Check sheet for the modelled part. Datum: model origin and axes. Units: mm. A direction names the side the tool comes from. Round coordinates to 2 decimals unless told otherwise and drop trailing zeros. Order: outer loops, then holes, each group sorted by start corner. A loop starts at its lowest first (then second) coordinate and runs counter-clockwise, first axis right, second up.
```python
from build123d import *

# Parameters (mm, degrees)
SKETCH1_W           = 10
SKETCH1_H           = 10
BOSS_EXTRUDE1_DEPTH = 5
SKETCH2_W           = 3
SKETCH2_H           = 5
CUT_EXTRUDE1_DEPTH  = 13.247448714
SKETCH3_W           = 3
SKETCH3_H           = 3
BOSS_EXTRUDE2_DEPTH = 5
SKETCH4_W           = 2
SKETCH4_H           = 2
BOSS_EXTRUDE3_DEPTH = 2


with BuildPart() as part:
    # Sketch1 → Boss-Extrude1 (new, symmetric)
    with BuildSketch(Plane(origin=(0, 0, 0), x_dir=(1, 0, 0), z_dir=(0, 1, 0))):
        Rectangle(SKETCH1_W, SKETCH1_H)
    extrude(amount=BOSS_EXTRUDE1_DEPTH, both=True)

    # Sketch2 → Cut-Extrude1 (cut, through all)
    with BuildSketch(Plane.XY.offset(5)):
        with Locations((-3.5, 0)):
            Rectangle(SKETCH2_W, SKETCH2_H)
    extrude(amount=-CUT_EXTRUDE1_DEPTH, mode=Mode.SUBTRACT)

    # Sketch3 → Boss-Extrude2 (add)
    with BuildSketch(Plane(origin=(5, 0, 0), x_dir=(0, 0, -1), z_dir=(1, 0, 0))):
        Rectangle(SKETCH3_W, SKETCH3_H)
    extrude(amount=BOSS_EXTRUDE2_DEPTH)

    # Sketch4 → Boss-Extrude3 (add)
    with BuildSketch(Plane(origin=(5, 0, 0), x_dir=(0, 0, -1), z_dir=(1, 0, 0))):
        with Locations((0, 4)):
            Rectangle(SKETCH4_W, SKETCH4_H)
    boss_extrude3 = extrude(amount=BOSS_EXTRUDE3_DEPTH)

    # Mirror1: Boss-Extrude3 across plane
    add(boss_extrude3.mirror(Plane.ZX))


solid = part.part
```
Item 1: Sectioned sample at B-B (y = -1). Record the cut outline in (x, z).
Answer:
outline: (-2, -5) - (5, -5) - (5, -1.5) - (10, -1.5) - (10, 1.5) - (5, 1.5) - (5, 5) - (-2, 5) - close
Item 2: Scan lines: line 1 along Y through (x, z) = (-2.75, -2); line 2 along X through (y, z) = (0.75, -3); line 3 along X through (y, z) = (-1, -1). Record each from-to range of solid material in increasing order.
Answer:
line 1: y = -5 to -2.5, 2.5 to 5
line 2: x = -2 to 5
line 3: x = -2 to 10
Item 3: Release check for a two-part mould opening along Y. For faces 5 (the flat face through (7, 4, 0)), 6 (the flat face through (7, -1.5, 0)), 7 (the flat face through (1, -5, 0)), 8 (the flat face through (1, 5, 0)) record: released by +Y, released by -Y, zero draft, split by the parting line, or undercut.
Answer:
face 5: zero draft
face 6: undercut
face 7: released by -Y
face 8: released by +Y
Item 4: Access from +Z, -Z, +X, -X, +Y, -Y to the whole of each face (thin tool, end or side, straight path). Record for faces 1 (the flat face through (6, 4, 1)), 2 (the flat face through (7, 0, -1.5)), 3 (the flat face through (7, 0, 1.5)), 4 (the flat face through (7, 1.5, 0)).
Answer:
face 1: +Z, +X, +Y
face 2: -Z, +X, +Y, -Y
face 3: +Z, +X, +Y, -Y
face 4: +Z, -Z, +X
Item 5: Go/stop test with flat-tipped pins: P1, Ø1.5, axis at x = 7, y = 0.5, coming from the +Z side; P2, Ø4, axis at y = 1, z = -1, coming from the -X side; P3, Ø1, axis at y = -3.5, z = 0.5, coming from the +X side; P4, Ø2.5, axis at x = 8, y = -0.5, coming from the -Z side. Record where each tip stops, or that it passes through.
Answer:
P1: stops at z = 1.5
P2: stops at x = -5
P3: stops at x = 7
P4: stops at z = -1.5
Item 6: Sectioned sample at D-D (z = 0.75). Record the cut outline in (x, y).
Answer:
outline: (-5, -5) - (7, -5) - (7, -3) - (5, -3) - (5, -1.5) - (10, -1.5) - (10, 1.5) - (5, 1.5) - (5, 3) - (7, 3) - (7, 5) - (-5, 5) - (-5, 2.5) - (-2, 2.5) - (-2, -2.5) - (-5, -2.5) - close
Item 7: Sectioned sample at A-A (z = -3.5). Record the cut outline in (x, y).
Answer:
outline: (-5, -5) - (5, -5) - (5, 5) - (-5, 5) - (-5, 2.5) - (-2, 2.5) - (-2, -2.5) - (-5, -2.5) - close
Item 8: Sectioned sample at C-C (x = 7.5). Record the cut outline in (y, z).
Answer:
outline: (-1.5, -1.5) - (1.5, -1.5) - (1.5, 1.5) - (-1.5, 1.5) - close
